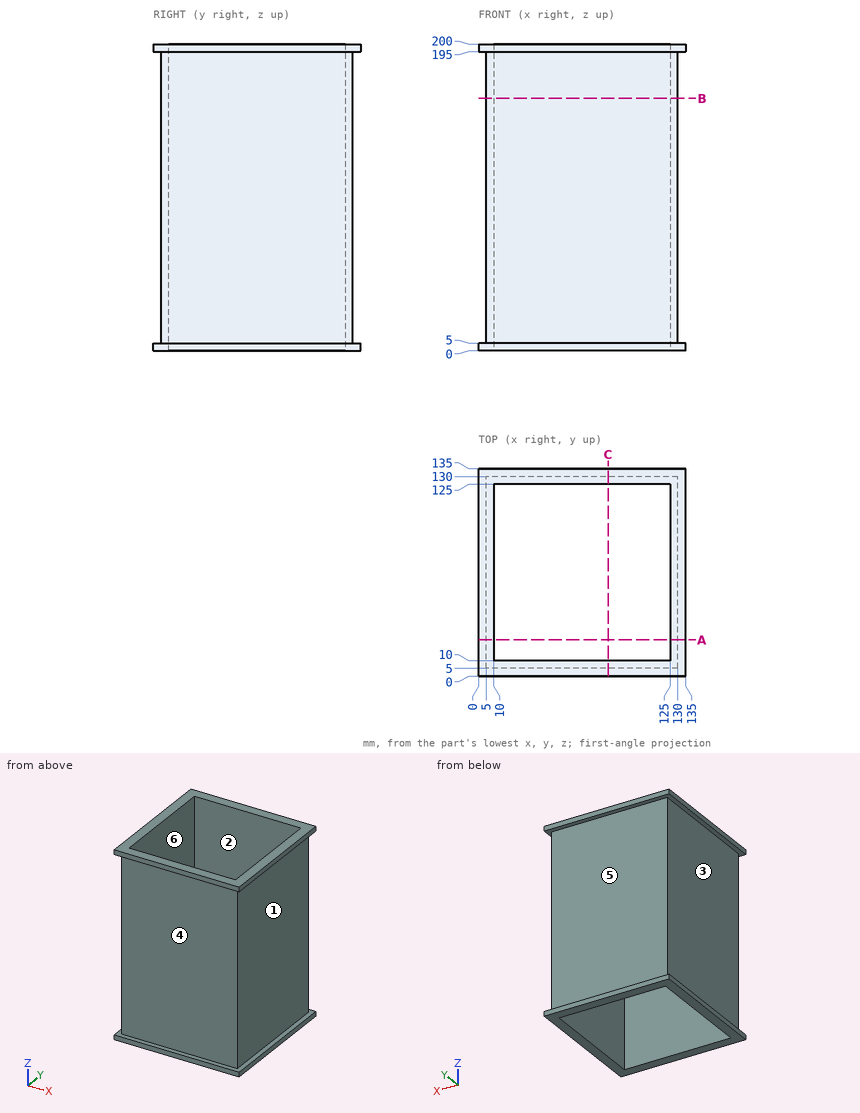
Part print with two shaded views. Sizes in mm from the minimum x, y, z corner. A direction names the side the tool comes from. Round coordinates to 2 decimals unless told otherwise and drop trailing zeros. Write each loop counter-clockwise with the first axis right and the second up, starting at its lowest first coordinate (ties: lowest second). Pieces come first, ordered by that corner, then holes. Notation, with made-up numbers: (7, 34.25) - (45, 34.25) arc R17 ccw to (45, 65.25) - close; hole circle Ø1 at (7, 34.5). An arc over 180 degrees is marked (long way). Answer as CSV lines item,"result".
Q1. Pull direction Z, two halves, no side cores. Call the marked faces 5 and 6: +Z half, -Z half, draft (parallel to the pull), parting line (faces both ways), or undercut.
Report:
face 5,"undercut"
face 6,"draft"
Q2. Drill centre line: probe 1 along X at (y, z) = (31, 129). Where is it in solid material? Low to high. Write a range as [from, to].
Report:
probe 1,"x = [5, 10], [125, 130]"
Q3. Cut at B-B (z = 164.5). Write the cut outline in (x, y).
Report:
outline,"(5, 5) - (130, 5) - (130, 130) - (5, 130) - close; hole (10, 10) - (125, 10) - (125, 125) - (10, 125) - close"
Q4. Drop flat-ended pins along their axis: pin 1 (1.5 mm diameter, centred on y = 108.5, z = 153.5, fed in from -X); pin 2 (1.5 mm diameter, centred on y = 17, z = 54, fed in from +X); pin 3 (8 mm diameter, centred on x = 78, z = 120, fed in from +Y). Give the stop position or say it passes through.
Report:
pin 1,"stops at x = 5"
pin 2,"stops at x = 130"
pin 3,"stops at y = 130"
Q5. Cut at A-A (y = 23.5). Write the cut outline in (x, z).
Report:
outline,"(0, 0) - (10, 0) - (10, 200) - (0, 200) - (0, 195) - (5, 195) - (5, 5) - (0, 5) - close; (125, 0) - (135, 0) - (135, 5) - (130, 5) - (130, 195) - (135, 195) - (135, 200) - (125, 200) - close"
Q6. Tool access for the marked faces 1, 2, 3 and 4: list every direction of +Z, -Z, +X, -X, +Y, -Y with a clear straight run to the whole face (end or side of a thin tool).
Report:
face 1,"+X, +Y, -Y"
face 2,"+Z, -Z"
face 3,"-X, +Y, -Y"
face 4,"+X, -X, -Y"
